from build123d import *

# Parameters (mm, degrees)
F1_DEPTH = 20
F2_W     = 9
F2_H     = 43
F3_DEPTH = 3
F4_DEPTH = 3
F5_R     = 2.99999


# Not quite as in the source:
# - a fillet or chamfer is up to 0.001 mm smaller than in the source, because OpenCascade refuses the exact size
# - a feature names something its author has since deleted; it is built from what else it names


with BuildPart() as f1:
    # F0 (on Top) → F1 (new body)
    with BuildSketch(Plane.XY):
        with BuildLine():
            Line((7.553949271, 11.7871900982), (9.1726526862, 14.3130165478))
            ThreePointArc((9.1726526862, 14.3130165478), (-4.0313436719, 16.5150921341), (-14.7357025028, 8.4769730299))
            Line((-14.7357025028, 8.4769730299), (-14.7357025028, -8.4769730299))
            ThreePointArc((-14.7357025028, -8.4769730299), (-4.0313436719, -16.5150921341), (9.1726526862, -14.3130165478))
            Line((9.1726526862, -14.3130165478), (7.553949271, -11.7871900982))
            ThreePointArc((7.553949271, -11.7871900982), (-14, 0), (7.553949271, 11.7871900982))
        make_face()
    extrude(amount=F1_DEPTH)

    # F2 (on face) → F3 (join)
    with BuildSketch(Plane(origin=(-14.7357025028, 0, 0), x_dir=(0, -1, 0), z_dir=(-1, 0, 0))):
        with Locations((0.0303052693, -1.5)):
            Rectangle(F2_W, F2_H)
    extrude(amount=F3_DEPTH)

    # F2 (on face) → F4 (join)
    with BuildSketch(Plane(origin=(-14.7357025028, 0, 0), x_dir=(0, -1, 0), z_dir=(-1, 0, 0))):
        with Locations((0.0303052693, -1.5)):
            Rectangle(F2_W, F2_H)
    extrude(amount=F4_DEPTH)

    # F5 (radius 3 in the source; OpenCascade refuses exactly that, so slightly less here)
    f5_edges = [f1.edges().sort_by_distance(p)[0] for p in [
        (-14.735703, 4.469695, 10),
        (-14.735703, -4.530305, 10),
    ]]
    fillet(f5_edges, radius=F5_R)


solid = f1.part
Work out the finished part from the listing and answer in its coordinate system (mm). A direction names the side the tool comes from. Round coordinates to 2 decimals unless told otherwise and drop trailing zeros. Write each loop counter-clockwise with the first axis right and the second up, starting at its lowest first coordinate (ties: lowest second). Pieces come first, ordered by that corner, then holes.
1) Straight lines are drawn through the part: line 1 (Y direction, x = 0, z = 14); line 2 (X direction, y = -1, z = -1); line 3 (X direction, y = 0, z = 7). For each, find the intervals that lie inside material, in ascending order.
2) A tool of negligible diameter and unlimited length cuts with its end or side. For faces 1 (the flat face through (-14.736, -8, 10)), 2 (the flat face through (-16, 4.47, -11)), 3 (the flat face through (8.35, 13.03, 9.86)), from which of +Z, -Z, +X, -X, +Y, -Y can it reach the whole face along a straight path? Write none if from no direction.
3) A cutting plane is placed at D-D (y = 0). Give the vertices of the cut face in (x, z).
4) The mould has two halves that part along Y. Classify faces 4 (the flat face through (8.375, -13.068, 9.86)), 5 (the flat face through (-16, -4.53, -11)), 6 (the flat face through (-13.3, -5, 0)): pulls with the +Y half, pulls with the -Y half, needs draft (parallel to the pull), parting line crosses it, or undercut.
5) A cutting plane is placed at C-C (y = 13.5). Give the vertices of the cut face in (x, z).
6) A cutting plane is placed at A-A (x = -7.5). Give the vertices of the cut face in (y, z).
7) Given pin 1 Ø4.5 at (y, z) = (-1.5, -16) entering from +X; pin 2 Ø1 at (x, z) = (5, 13.5) entering from -Y; pin 3 Ø1 at (y, z) = (-8, 5.5) entering from -X, each flat-ended and moving along its own axis, determine where each tip first touches the part or whether it passes through.
Completed:
1. line 1: y = -17 to -14, 14 to 17
1. line 2: x = -17.74 to -14.74
1. line 3: x = -17.74 to -14
2. face 1: +Z, -Z, -X, -Y
2. face 2: -Z, +X, -X, +Y
2. face 3: +Z, -Z, +X
3. outline: (-17.74, -23) - (-14.74, -23) - (-14.74, 0) - (-14, 0) - (-14, 20) - (-17.74, 20) - close
4. face 4: undercut
4. face 5: pulls with the -Y half
4. face 6: needs draft
5. outline: (-10.33, 0) - (-3.71, 0) - (-3.71, 20) - (-10.33, 20) - close; (3.71, 0) - (8.65, 0) - (8.65, 20) - (3.71, 20) - close
6. outline: (-15.26, 0) - (-11.82, 0) - (-11.82, 20) - (-15.26, 20) - close; (11.82, 0) - (15.26, 0) - (15.26, 20) - (11.82, 20) - close
7. pin 1: stops at x = -14.74
7. pin 2: stops at y = -16.39
7. pin 3: stops at x = -14.74
